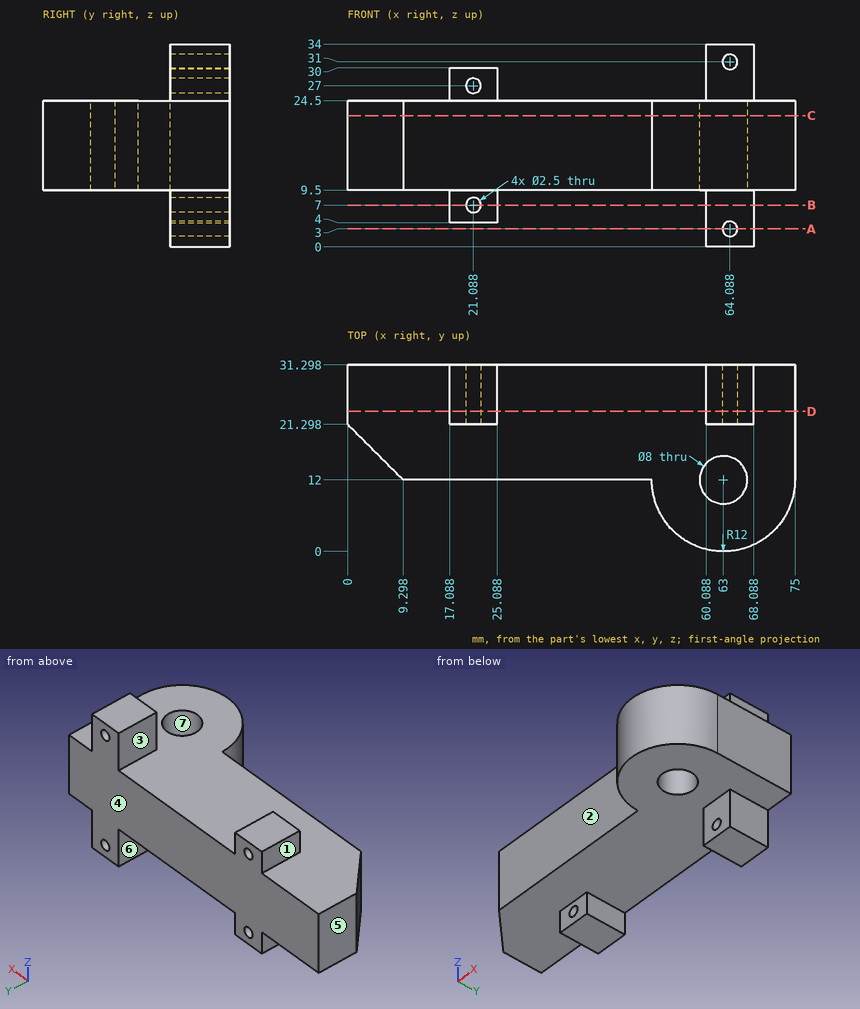
Job drawing, mm, ordinate dimensions from the low corner. One solid piece. A direction names the side the tool comes from. Give positions to 0.01 mm unless a question says otherwise; leave off trailing zeros. Loops run counter-clockwise (first coordinate to the right, second up) from the corner with the lowest first, then second, coordinate; pieces in that order, holes last. Notation, with made-up numbers: (82.25, 65) -> (108.25, 65) arc R3 cw to (108.25, 70) -> close; hole circle Ø4 at (-29.5, 50). An arc over 180 degrees is marked (long way). Write each question's results on one line, items separated by ' | '.
(1) Tool access for the marked faces 1, 2 and 3: list every direction of +Z, -Z, +X, -X, +Y, -Y with a clear straight run to the whole face (end or side of a thin tool).
Geometry results:
face 1: +Z, -X, +Y, -Y | face 2: +Z, -Z, -X, -Y | face 3: +Z, +Y, -Y
(2) Pull direction X, two halves, no side cores. Call the marked faces 4, 5, 6 and 7: released by +X, released by -X, zero draft, split by the parting line, or undercut.
Geometry results:
face 4: zero draft | face 5: released by -X | face 6: undercut | face 7: undercut
(3) Flat gauge pins, fed straight in: pin 1 Ø2.5 at (x, z) = (63, 5) entering from -Y; pin 2 Ø3 at (x, z) = (21.09, 27) entering from +Y; pin 3 Ø2 at (x, y) = (26.5, 14.5) entering from +Z; pin 4 Ø9.5 at (x, y) = (24.5, 17.5) entering from +Z. Where does each tip first touch, or does it go through?
Geometry results:
pin 1: stops at y = 21.3 | pin 2: stops at y = 31.3 | pin 3: stops at z = 24.5 | pin 4: stops at z = 30
(4) Cut at A-A on z = 3. List the corners of the cut face in (x, y), and give its area (3 significant figures).
Geometry results:
outline: (60.09, 21.3) -> (62.84, 21.3) -> (62.84, 31.3) -> (60.09, 31.3) -> close; (65.34, 21.3) -> (68.09, 21.3) -> (68.09, 31.3) -> (65.34, 31.3) -> close | area: 55.0 mm²
(5) Cut at C-C on z = 22. List the corners of the cut face in (x, y).
Geometry results:
outline: (0, 21.3) -> (9.3, 12) -> (51, 12) arc R12 ccw to (75, 12) -> (75, 31.3) -> (0, 31.3) -> close; hole circle Ø8 at (63, 12)
(6) Probe line 1 along X through (y, z) = (28, 5); line 2 along Z through (x, y) = (6, 24); line 3 along Y through (x, z) = (61, 8.5). List the from-to ranges inside material, lowest first.
Geometry results:
line 1: x = 17.09 to 25.09, 60.09 to 68.09 | line 2: z = 9.5 to 24.5 | line 3: y = 21.3 to 31.3
(7) Cut at D-D on y = 23.5. List the corners of the cut face in (x, z), and give its area (3 significant figures).
Geometry results:
outline: (0, 9.5) -> (17.09, 9.5) -> (17.09, 4) -> (25.09, 4) -> (25.09, 9.5) -> (60.09, 9.5) -> (60.09, 0) -> (68.09, 0) -> (68.09, 9.5) -> (75, 9.5) -> (75, 24.5) -> (68.09, 24.5) -> (68.09, 34) -> (60.09, 34) -> (60.09, 24.5) -> (25.09, 24.5) -> (25.09, 30) -> (17.09, 30) -> (17.09, 24.5) -> (0, 24.5) -> close; hole circle Ø2.5 at (21.09, 7); hole circle Ø2.5 at (21.09, 27); hole circle Ø2.5 at (64.09, 3); hole circle Ø2.5 at (64.09, 31) | area: 1,350 mm²
(8) Cut at B-B on z = 7. List the corners of the cut face in (x, y), and give its area (3 significant figures).
Geometry results:
outline: (17.09, 21.3) -> (19.84, 21.3) -> (19.84, 31.3) -> (17.09, 31.3) -> close; (22.34, 21.3) -> (25.09, 21.3) -> (25.09, 31.3) -> (22.34, 31.3) -> close; (60.09, 21.3) -> (68.09, 21.3) -> (68.09, 31.3) -> (60.09, 31.3) -> close | area: 135 mm²
